from build123d import *

# Parameters (mm, degrees)
BOSS_EXTRUDE1_DEPTH = 4
CUT_EXTRUDE2_DEPTH  = 1
SKETCH5_R           = 2
CUT_EXTRUDE3_DEPTH  = 22.132971525
CUT_EXTRUDE4_DEPTH  = 22.132971525
SKETCH7_W           = 18.4
SKETCH7_H           = 2
BOSS_EXTRUDE2_DEPTH = 10
SKETCH8_R           = 1.5
CUT_EXTRUDE5_DEPTH  = 25.154392176


with BuildPart() as part:
    # Sketch1 → Boss-Extrude1 (new body)
    with BuildSketch(Plane(origin=(0, 0, 0), x_dir=(1, 0, 0), z_dir=(0, 1, 0))):
        with BuildLine():
            Line((-12.649074074, 14.633101852), (5.750925926, 14.633101852))
            ThreePointArc((5.750925926, 14.633101852), (7.377271523, 13.959447449), (8.050925926, 12.333101852))
            Line((8.050925926, 12.333101852), (8.050925926, -6.566898148))
            ThreePointArc((8.050925926, -6.566898148), (7.377271523, -8.193243745), (5.750925926, -8.866898148))
            Line((5.750925926, -8.866898148), (-12.649074074, -8.866898148))
            ThreePointArc((-12.649074074, -8.866898148), (-14.275419671, -8.193243745), (-14.949074074, -6.566898148))
            Line((-14.949074074, -6.566898148), (-14.949074074, 12.333101852))
            ThreePointArc((-14.949074074, 12.333101852), (-14.275419671, 13.959447449), (-12.649074074, 14.633101852))
        make_face()
    extrude(amount=BOSS_EXTRUDE1_DEPTH)

    # Sketch2 → Cut-Extrude2 (cut)
    with BuildSketch(Plane(origin=(0, 4, 0), x_dir=(1, 0, 0), z_dir=(0, 1, 0))):
        with BuildLine():
            Line((5.750925926, 13.633101852), (-12.649074074, 13.633101852))
            ThreePointArc((-12.649074074, 13.633101852), (-13.56831289, 13.252340667), (-13.949074074, 12.333101852))
            Line((-13.949074074, 12.333101852), (-13.949074074, -6.566898148))
            ThreePointArc((-13.949074074, -6.566898148), (-13.56831289, -7.486136964), (-12.649074074, -7.866898148))
            Line((-12.649074074, -7.866898148), (5.750925926, -7.866898148))
            ThreePointArc((5.750925926, -7.866898148), (6.670164741, -7.486136964), (7.050925926, -6.566898148))
            Line((7.050925926, -6.566898148), (7.050925926, 12.333101852))
            ThreePointArc((7.050925926, 12.333101852), (6.670164741, 13.252340667), (5.750925926, 13.633101852))
        make_face()
    extrude(amount=-CUT_EXTRUDE2_DEPTH, mode=Mode.SUBTRACT)

    # Sketch5 → Cut-Extrude3 (cut, through all)
    with BuildSketch(Plane(origin=(0, 3, 0), x_dir=(1, 0, 0), z_dir=(0, 1, 0))):
        with Locations(Location((5.050925926, 11.633101852, 0), (0, 0, 270))):
            Circle(SKETCH5_R)
        with Locations(Location((5.050925926, -5.866898148, 0), (0, 0, 270))):
            Circle(SKETCH5_R)
        with Locations(Location((-11.949074074, -5.866898148, 0), (0, 0, 270))):
            Circle(SKETCH5_R)
        with Locations(Location((-11.949074074, 11.633101852, 0), (0, 0, 90))):
            Circle(SKETCH5_R)
    extrude(amount=-CUT_EXTRUDE3_DEPTH, mode=Mode.SUBTRACT)

    # Sketch6 → Cut-Extrude4 (cut, through all)
    with BuildSketch(Plane(origin=(0, 3, 0), x_dir=(1, 0, 0), z_dir=(0, 1, 0))):
        with BuildLine():
            Line((4.050925926, -3.038471023), (4.050925926, 8.804674727))
            ThreePointArc((4.050925926, 8.804674727), (2.601436183, 9.901051044), (2.050925926, 11.633101852))
            Line((2.050925926, 11.633101852), (2.050925926, -5.866898148))
            ThreePointArc((2.050925926, -5.866898148), (2.601436183, -4.134847341), (4.050925926, -3.038471023))
        make_face()
        with BuildLine():
            Line((-10.949074074, 8.804674727), (-10.949074074, -3.038471023))
            ThreePointArc((-10.949074074, -3.038471023), (-9.499584331, -4.134847341), (-8.949074074, -5.866898148))
            Line((-8.949074074, -5.866898148), (-8.949074074, 11.633101852))
            ThreePointArc((-8.949074074, 11.633101852), (-9.499584331, 9.901051044), (-10.949074074, 8.804674727))
        make_face()
    extrude(amount=-CUT_EXTRUDE4_DEPTH, mode=Mode.SUBTRACT)

    # Sketch7 → Boss-Extrude2 (add)
    with BuildSketch(Plane.XY.offset(8.866898148)):
        with Locations((-3.449074074, 1)):
            Rectangle(SKETCH7_W, SKETCH7_H)
    extrude(amount=BOSS_EXTRUDE2_DEPTH)

    # Sketch8 → Cut-Extrude5 (cut, through all)
    with BuildSketch(Plane(origin=(0, 2, 0), x_dir=(1, 0, 0), z_dir=(0, 1, 0))):
        with Locations(Location((1.150925926, -13.866898148, 0), (0, 0, 270))):
            Circle(SKETCH8_R)
        with Locations(Location((-8.049074074, -13.866898148, 0), (0, 0, 270))):
            Circle(SKETCH8_R)
    extrude(amount=-CUT_EXTRUDE5_DEPTH, mode=Mode.SUBTRACT)


solid = part.part
Could you check a few things on this model? Use its own coordinates, in mm. A direction names the side the tool comes from. Give positions to 0.01 mm unless a question says otherwise; leave off trailing zeros. Write each loop counter-clockwise with the first axis right and the second up, starting at its lowest first coordinate (ties: lowest second). Pieces come first, ordered by that corner, then holes. Notation, with made-up numbers: (11.5, -6.5) -> (43.5, -6.5) arc R14 cw to (43.5, 7.5) -> close; hole circle Ø9 at (63.25, 47). An arc over 180 degrees is marked (long way). Write each question's results on one line, items separated by ' | '. Start each with the question number.
Q1. Suppose I cut it at B-B, the plane y = 2.35. List the corners of the cut face in (x, z) for me.
Q2. Suppose I cut it at A-A, the plane z = -6. List the corners of the cut face in (x, y) for me, and give its area (3 significant figures).
Q3. Suppose I cut it at D-D, the plane z = -11. List the corners of the cut face in (x, y) for me.
Q4. I need wall thicknesses on probe 1 along X at (y, z) = (2.6, -3); probe 2 along Z at (x, y) = (6, 0.85); probe 3 along X at (y, z) = (0.2, 7). Which ranges of each line are inside material? Lowest first, please.
Q5. I'm going to push flat-ended pins straight in: pin 1 Ø5 at (x, z) = (-0.5, 14) entering from +Y; pin 2 Ø1.6 at (x, y) = (-7, 3) entering from +Z; pin 3 Ø1 at (y, z) = (1, 14) entering from -X. Where does each tip first touch, or does it pass through?
Q6. Suppose I cut it at C-C, the plane x = -11.5. List the corners of the cut face in (y, z) for me, and give its area (3 significant figures).
Q7. Which directions (+Z, -Z, +X, -X, +Y, -Y) give clear straight access to the entire face, cutting with the end or side of a thin tool? Please do faces 1 (the face through (7.395, 1.972, 8.175)), 2 (the face through (4.051, 2, -3)), 3 (the face through (-4, 3, -3)).
Outcome:
1) outline: (-14.95, -12.33) arc R2.3 ccw to (-12.65, -14.63) -> (5.75, -14.63) arc R2.3 ccw to (8.05, -12.33) -> (8.05, 6.57) arc R2.3 ccw to (5.75, 8.87) -> (-12.65, 8.87) arc R2.3 ccw to (-14.95, 6.57) -> close; hole circle Ø4 at (-11.95, -11.63); hole circle Ø4 at (-11.95, 5.87); hole (-10.95, -8.8) arc R3 cw to (-8.95, -11.63) -> (-8.95, 5.87) arc R3 cw to (-10.95, 3.04) -> close; hole (2.05, -11.63) arc R3 cw to (4.05, -8.8) -> (4.05, 3.04) arc R3 cw to (2.05, 5.87) -> close; hole circle Ø4 at (5.05, -11.63); hole circle Ø4 at (5.05, 5.87)
2) outline: (-14.95, 0) -> (-10.95, 0) -> (-10.95, 3) -> (-13.95, 3) -> (-13.95, 4) -> (-14.95, 4) -> close; (-8.95, 0) -> (2.05, 0) -> (2.05, 3) -> (-8.95, 3) -> close; (4.05, 0) -> (8.05, 0) -> (8.05, 4) -> (7.05, 4) -> (7.05, 3) -> (4.05, 3) -> close | area: 59.0 mm2
3) outline: (-14.95, 0) -> (-13.85, 0) -> (-13.85, 3) -> (-13.95, 3) -> (-13.95, 4) -> (-14.95, 4) -> close; (-10.05, 0) -> (-9.02, 0) -> (-9.02, 3) -> (-10.05, 3) -> close; (-8.95, 0) -> (2.05, 0) -> (2.05, 3) -> (-8.95, 3) -> close; (2.12, 0) -> (3.15, 0) -> (3.15, 3) -> (2.12, 3) -> close; (6.95, 0) -> (8.05, 0) -> (8.05, 4) -> (7.05, 4) -> (7.05, 3) -> (6.95, 3) -> close
4) probe 1: -14.95 to -10.95, -8.95 to 2.05, 4.05 to 8.05 | probe 2: -14.62 to -13.39, -9.87 to 4.11, 7.63 to 8.85 | probe 3: -14.91 to -13.6, -10.3 to 3.4, 6.7 to 8.01
5) pin 1: y = 2 | pin 2: z = 8.87 | pin 3: x = -12.65
6) outline: (0, -14.63) -> (4, -14.63) -> (4, -13.63) -> (3, -13.63) -> (3, -13.58) -> (0, -13.58) -> close; (0, -9.68) -> (3, -9.68) -> (3, 3.92) -> (0, 3.92) -> close; (0, 7.82) -> (3, 7.82) -> (3, 7.87) -> (4, 7.87) -> (4, 8.87) -> (2, 8.87) -> (2, 18.87) -> (0, 18.87) -> close | area: 69.1 mm2
7) face 1: +Z, +X, +Y, -Y | face 2: +Y, -Y | face 3: +Y
